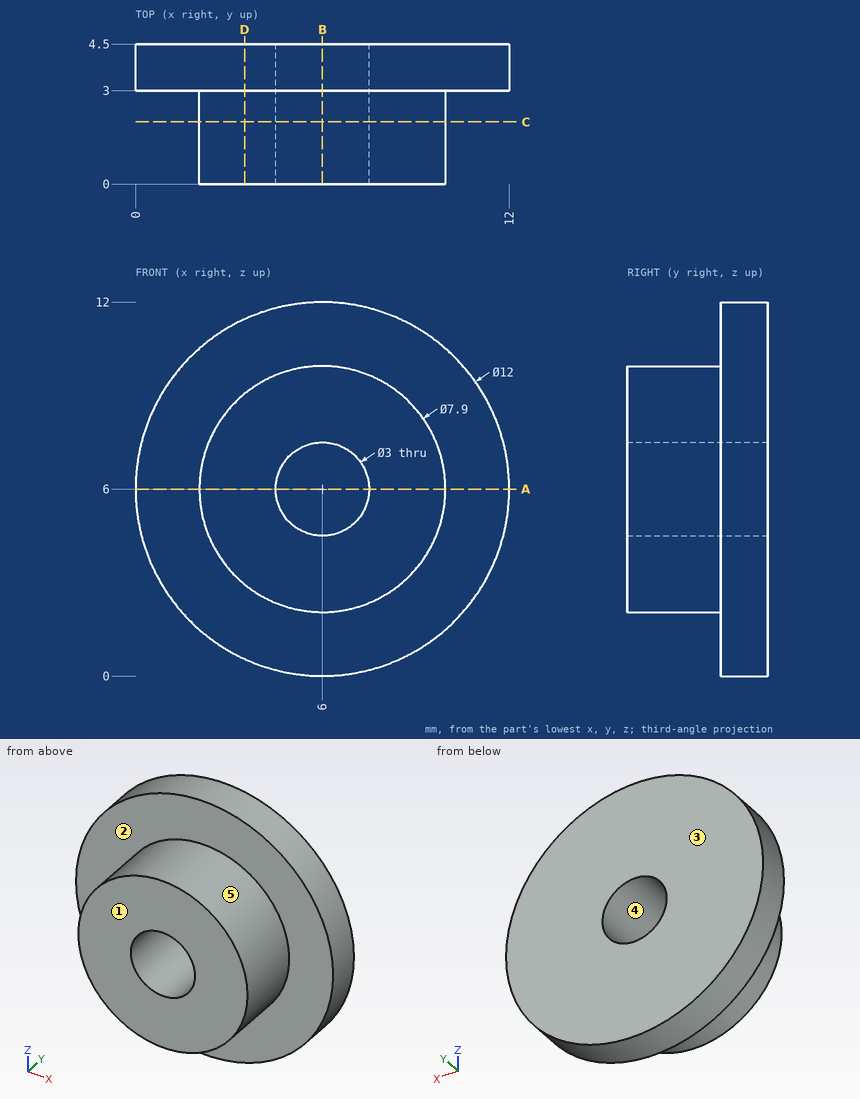
Answer from the drawing. Dimensions are ordinates in mm from the lowest x, y and z of the part. A direction names the side the tool comes from. Give positions to 0.01 mm unless a question says otherwise; leave off trailing zeros. Loops run counter-clockwise (first coordinate to the right, second up) from the corner with the lowest first, then second, coordinate; pieces in that order, holes last. Notation, with made-up numbers: M -8.5,23 L 34.5,23 A19 ccw 34.5,56 Z; hole C 81,-15 d11. An arc over 180 degrees is marked long. One line per item, written item: value.
Q1. A cutting plane is placed at A-A on z = 6. Determine the outline of the cut face in (x, y), then the cut area to 3 significant figures.
Working result:
outline: M 0,3 L 2.05,3 L 2.05,0 L 4.5,0 L 4.5,4.5 L 0,4.5 Z; M 7.5,0 L 9.95,0 L 9.95,3 L 12,3 L 12,4.5 L 7.5,4.5 Z
area: 28.2 mm^2
Q2. A cutting plane is placed at B-B on x = 6. Determine the outline of the cut face in (y, z).
Working result:
outline: M 0,2.05 L 3,2.05 L 3,0 L 4.5,0 L 4.5,4.5 L 0,4.5 Z; M 0,7.5 L 4.5,7.5 L 4.5,12 L 3,12 L 3,9.95 L 0,9.95 Z
Q3. For the marked faces 1 and 2, determine the directions among +Z, -Z, +X, -X, +Y, -Y from which every point of the face is accessible in a straight line to the end or side of a thin tool.
Working result:
face 1: +Z, -Z, +X, -X, -Y
face 2: -Y
Q4. Find the intervals of material crossed by line 1 (Z direction, x = 6, y = 2.65); line 2 (Z direction, x = 6, y = 3.15); line 3 (Y direction, x = 4.25, z = 10.5), in increasing order. Write a range as from..to.
Working result:
line 1: z = 2.05..4.5, 7.5..9.95
line 2: z = 0..4.5, 7.5..12
line 3: y = 3..4.5
Q5. A cutting plane is placed at D-D on x = 3.5. Determine the outline of the cut face in (y, z), then the cut area to 3 significant figures.
Working result:
outline: M 0,2.94 L 3,2.94 L 3,0.55 L 4.5,0.55 L 4.5,11.45 L 3,11.45 L 3,9.06 L 0,9.06 Z
area: 34.7 mm^2
Q6. Flat-ended cylindrical pins translate along their axes: P1, Ø2, axis at x = 4.5, y = 3, coming from the -Z side; P2, Ø1.5, axis at x = 10, z = 10, coming from the -Y side; P3, Ø1.5, axis at x = 9, y = 1, coming from the -Z side. Find the tip coordinate at first contact, or state that the pin passes through.
Working result:
P1: stops at z = 0.02
P2: stops at y = 3
P3: stops at z = 2.75
Q7. A cutting plane is placed at C-C on y = 2. Determine the outline of the cut face in (x, z).
Working result:
outline: C 6,6 d7.9; hole C 6,6 d3
Q8. Determine the mould class of the marked faces 3, 4 and 5 for opening direction Z: +Z half, -Z half, draft (parallel to the pull), parting line (faces both ways), or undercut.
Working result:
face 3: draft
face 4: undercut
face 5: parting line
